Check sheet for the modelled part. Datum: model origin and axes. Units: mm. Coordinates: 2 decimals unless noted, no trailing zeros. Loops run counter-clockwise (first coordinate to the right, second up) from the corner with the lowest first, then second, coordinate; pieces in that order, holes last. Notation, with made-up numbers: (65, 12.25) -> (124, 12.25) arc R22 ccw to (124, 39.25) -> close; hole circle Ø7 at (-9, 57). An arc over 180 degrees is marked (long way). Use one line per item in the form item = value.
from build123d import *

# Parameters (mm, degrees)
SKETCH_1_R          = 45
EXTRUDE_1_DEPTH     = 12
SKETCH_5_R          = 2
CUT_EXTRUDE_1_DEPTH = 20
SKETCH_6_R          = 2
CUT_EXTRUDE_2_DEPTH = 21


with BuildPart() as part:
    # 草图1 → 凸台-拉伸1 (new body)
    with BuildSketch(Plane.XY):
        Circle(SKETCH_1_R)
    extrude(amount=EXTRUDE_1_DEPTH)

    # 草图5 → 切除-拉伸1 (cut)
    with BuildSketch(Plane(origin=(0, 0, 0), x_dir=(-1, 0, 0), z_dir=(0, 0, -1))):
        with Locations((-15.476254719, 7.618926425)):
            Circle(SKETCH_5_R)
        with Locations((-1.139943526, 17.212292955)):
            Circle(SKETCH_5_R)
        with Locations((14.336311193, 9.59336653)):
            Circle(SKETCH_5_R)
        with Locations((15.476254719, -7.618926425)):
            Circle(SKETCH_5_R)
        with Locations((1.139943526, -17.212292955)):
            Circle(SKETCH_5_R)
        with Locations((-14.336311193, -9.59336653)):
            Circle(SKETCH_5_R)
    extrude(amount=-CUT_EXTRUDE_1_DEPTH, mode=Mode.SUBTRACT)

    # 草图6 → 切除-拉伸2 (cut)
    with BuildSketch(Plane(origin=(0, 0, 0), x_dir=(-1, 0, 0), z_dir=(0, 0, -1))):
        Circle(SKETCH_6_R)
    extrude(amount=-CUT_EXTRUDE_2_DEPTH, mode=Mode.SUBTRACT)


solid = part.part
(1) Scan lines: line 1 along Y through (x, z) = (14, 10); line 2 along Y through (x, z) = (1.5, 4.5) (3 decimals); line 3 along X through (y, z) = (-18.5, 3.75). Record each from-to range of solid material in increasing order.
Established:
line_1 = -42.77 to -11.56, -7.62 to 6.27, 8.97 to 42.77
line_2 = -44.975 to -1.323, 1.323 to 15.245, 19.18 to 44.975
line_3 = -41.02 to -2.67, 0.39 to 41.02
(2) Go/stop test with flat-tipped pins: P1, Ø5, axis at x = 8, z = 5, coming from the -Y side; P2, Ø1, axis at y = -22.5, z = 4.5, coming from the +X side; P3, Ø3.5, axis at x = -14.34, y = 9.59, coming from the -Z side; P4, Ø5, axis at x = 26, z = 6, coming from the +Y side. Record where each tip stops, or that it passes through.
Established:
P1 = -44.66
P2 = 39.26
P3 = through
P4 = 38.38
(3) Section check A-A, the plane y = 0. Record the boundary of the cut face in (x, z).
Established:
outline = (-45, 0) -> (-2, 0) -> (-2, 12) -> (-45, 12) -> close; (2, 0) -> (45, 0) -> (45, 12) -> (2, 12) -> close
(4) Mould release check, pull along Y, two halves, no side actions. Record for faces 1 (the cylindrical face through (14.77, -11.546, 5.916)), 2 (the cylindrical face through (20.765, -39.923, 5.916)), 3 (the cylindrical face through (0, -2, 6)), 4 (the flat face through (-1, -9, 12)): +Y half, -Y half, draft (parallel to the pull), parting line (faces both ways), or undercut.
Established:
face_1 = undercut
face_2 = parting line
face_3 = undercut
face_4 = draft
(5) Section check B-B, the plane z = 8. Record the boundary of the cut face in (x, y), plus the area to 3 significant figures.
Established:
outline = circle Ø90 at (0, 0); hole circle Ø4 at (-15.48, -7.62); hole circle Ø4 at (-14.34, 9.59); hole circle Ø4 at (-1.14, -17.21); hole circle Ø4 at (0, 0); hole circle Ø4 at (1.14, 17.21); hole circle Ø4 at (14.34, -9.59); hole circle Ø4 at (15.48, 7.62)
area = 6,270 mm²
(6) Section check D-D, the plane x = -8. Record the boundary of the cut face in (y, z), plus the area to 3 significant figures.
Established:
outline = (-44.28, 0) -> (44.28, 0) -> (44.28, 12) -> (-44.28, 12) -> close
area = 1,060 mm²
(7) Section check C-C, the plane y = -36. Record the boundary of the cut face in (x, z), plus the area to 3 significant figures.
Established:
outline = (-27, 0) -> (27, 0) -> (27, 12) -> (-27, 12) -> close
area = 648 mm²
